Part model, mm, in its own coordinate system. Coordinates: 2 decimals unless noted, no trailing zeros. Write each loop counter-clockwise with the first axis right and the second up, starting at its lowest first coordinate (ties: lowest second). Pieces come first, ordered by that corner, then holes. Notation, with made-up numbers: (85, 65.25) -> (99, 65.25) arc R27 ccw to (99, 89.25) -> close; hole circle Ø7 at (20.5, -21). An arc over 180 degrees is marked (long way). Write item = value, one per line. Start each with the question number.
Q1. Probe line 1 (X direction, y = 1.8, z = -46.5); line 2 (X direction, y = 0.95, z = -48); line 3 (Z direction, x = 14, y = 2.1). List the from-to ranges inside material, lowest first.
Q2. Pin check, flat tip, straight feed: P1, Ø5.5, axis at x = 11.5, z = 46.5, coming from the -Y side. Stop position of the tip, or through.
Q3. Pull direction Z, two halves, no side cores. Call faces 1 (the cylindrical face through (-12.41, 1.52, -48.55)), 2 (the flat face through (0, 3, -2)), 3 (the cylindrical face through (23, 2, -109)): released by +Z, released by -Z, zero draft, split by the parting line, or undercut.
Q4. Band-saw the part on A-A, the plane y = 2.4. Give the number of separate pieces and of enclosed holes in the cut face, plus the area to 3 significant figures.
Q5. Band-saw the part on B-B, the plane z = -28.5. List the corners of the cut face in (x, y), plus the area to 3 significant figures.
from build123d import *

# Parameters (mm, degrees)
SKETCH1_W       = 50
SKETCH1_H       = 220
EXTRUDE1_DEPTH  = 3
SKETCH2_R       = 1.75
EXTRUDE2_DEPTH  = 3
SKETCH3_R       = 2.05
EXTRUDE3_DEPTH  = 3
SKETCH4_R       = 1.55
EXTRUDE4_DEPTH  = 3
LPATTERN1_COUNT = 2
LPATTERN1_PITCH = 210
LPATTERN2_COUNT = 2
LPATTERN2_PITCH = 75
FILLET1_R       = 5


with BuildPart() as part:
    # Sketch1 → Extrude1 (new body)
    with BuildSketch(Plane(origin=(0, 0, 0), x_dir=(1, 0, 0), z_dir=(0, 1, 0))):
        Rectangle(SKETCH1_W, SKETCH1_H)
    extrude(amount=EXTRUDE1_DEPTH)

    # Sketch2 → Extrude2 (cut)
    with BuildSketch(Plane(origin=(0, 3, 0), x_dir=(1, 0, 0), z_dir=(0, 1, 0))):
        with Locations(Location((20, 105, 0), (0, 0, 270))):
            Circle(SKETCH2_R)
    extrude2 = extrude(amount=-EXTRUDE2_DEPTH, mode=Mode.SUBTRACT)

    # Sketch3 → Extrude3 (cut)
    with BuildSketch(Plane(origin=(0, 3, 0), x_dir=(1, 0, 0), z_dir=(0, 1, 0))):
        with Locations(Location((-12.5, 46.5, 0), (0, 0, 270))):
            Circle(SKETCH3_R)
        with Locations(Location((11.5, 46.5, 0), (0, 0, 270))):
            Circle(SKETCH3_R)
        with Locations(Location((-12.5, 28.5, 0), (0, 0, 270))):
            Circle(SKETCH3_R)
        with Locations(Location((11.5, 28.5, 0), (0, 0, 270))):
            Circle(SKETCH3_R)
    extrude3 = extrude(amount=-EXTRUDE3_DEPTH, mode=Mode.SUBTRACT)

    # Sketch4 → Extrude4 (cut)
    with BuildSketch(Plane(origin=(0, 3, 0), x_dir=(1, 0, 0), z_dir=(0, 1, 0))):
        with Locations(Location((15, 10, 0), (0, 0, 270))):
            Circle(SKETCH4_R)
        with Locations(Location((15, -10, 0), (0, 0, 270))):
            Circle(SKETCH4_R)
        with Locations(Location((-10, 0, 0), (0, 0, 270))):
            Circle(SKETCH4_R)
    extrude(amount=-EXTRUDE4_DEPTH, mode=Mode.SUBTRACT)

    # LPattern1: Extrude2 ×2
    with Locations(*[(0, 0, i * LPATTERN1_PITCH) for i in range(1, LPATTERN1_COUNT)]):
        add(extrude2, mode=Mode.SUBTRACT)

    # LPattern2: Extrude3 ×2
    with Locations(*[(0, 0, i * LPATTERN2_PITCH) for i in range(1, LPATTERN2_COUNT)]):
        add(extrude3, mode=Mode.SUBTRACT)

    # Fillet1
    fillet1_edges = [part.edges().sort_by_distance(p)[0] for p in [
        (-25, 1.5, -110),
        (25, 1.5, -110),
        (25, 1.5, 110),
        (-25, 1.5, 110),
    ]]
    fillet(fillet1_edges, radius=FILLET1_R)


solid = part.part
Ans:
q1.line_1 = -25 to -14.55, -10.45 to 9.45, 13.55 to 25
q1.line_2 = -25 to -13.9, -11.1 to 10.1, 12.9 to 25
q1.line_3 = -110 to -11.18, -8.82 to 8.82, 11.18 to 110
q2.P1 = 0
q3.face_1 = undercut
q3.face_2 = zero draft
q3.face_3 = released by -Z
q4.separate_pieces = 1
q4.enclosed_holes = 13
q4.area = 10,800 mm2
q5.outline = (-25, 0) -> (-14.55, 0) -> (-14.55, 3) -> (-25, 3) -> close; (-10.45, 0) -> (9.45, 0) -> (9.45, 3) -> (-10.45, 3) -> close; (13.55, 0) -> (25, 0) -> (25, 3) -> (13.55, 3) -> close
q5.area = 125 mm2
